Check sheet for the modelled part. Datum: model origin and axes. Units: mm. Face numbers are marked on the shaded views. A direction names the side the tool comes from. Give positions to 0.01 mm unless a question says otherwise; leave off trailing zeros. Write each loop counter-clockwise with the first axis right and the second up, starting at its lowest first coordinate (ties: lowest second). Pieces come first, ordered by that corner, then holes. Notation, with made-up numbers: M -8,11.5 L 10,11.5 A13 ccw 10,28.5 Z; hole C 33.5,-23 d2. An arc over 180 degrees is marked long. Use CSV: the item, a comma, the result in double quotes. Start each with the question number.
1. Depth check by flat-ended pin: P1, Ø2, axis at x = -4.5, z = 5, coming from the -Y side; P2, Ø4, axis at x = -3.5, z = 2.5, coming from the +Y side. Enter the tip coordinate at first touch or a pass-through.
2. Cross-section at A-A, the plane y = 0.5. Enter the section's corners in (x, z), and give its area (3 significant figures).
3. Access from +Z, -Z, +X, -X, +Y, -Y to the whole of each face (thin tool, end or side, straight path). Record for the marked faces 4 and 5.
4. Mould release check, pull along Z, two halves, no side actions. Record for the marked faces 1, 2 and 3: +Z half, -Z half, draft (parallel to the pull), parting line (faces both ways), or undercut.
5. Cross-section at D-D, the plane y = 1.25. Enter the section's corners in (x, z).
6. Cross-section at C-C, the plane z = 5.75. Enter the section's corners in (x, y), and give its area (3 significant figures).
7. Scan lines: line 1 (Z direction, x = -4.5, y = 1); line 2 (X direction, y = 2, z = 4); line 3 (Z direction, x = -6, y = 1.75). Record each from-to range of solid material in increasing order.
8. Cross-section at B-B, the plane x = -4.75. Enter the section's corners in (y, z).
from build123d import *

# Parameters (mm, degrees)
BOSS_EXTRUDE1_DEPTH = 7.8
SHELL1_T            = -1.5


with BuildPart() as part:
    # Sketch1 → Boss-Extrude1 (new body)
    with BuildSketch(Plane(origin=(0, 0, 0), x_dir=(0, 0, -1), z_dir=(1, 0, 0))):
        Polygon((0, 0), (-7.8, 0), (-7.8, 2), (0, 6.15), align=None)
    extrude(amount=-BOSS_EXTRUDE1_DEPTH)

    # Shell1
    shell1_openings = [part.faces().sort_by_distance(p)[0] for p in [
        (-3.9, 0, 3.9),
    ]]
    offset(amount=SHELL1_T, openings=shell1_openings, kind=Kind.INTERSECTION)


solid = part.part
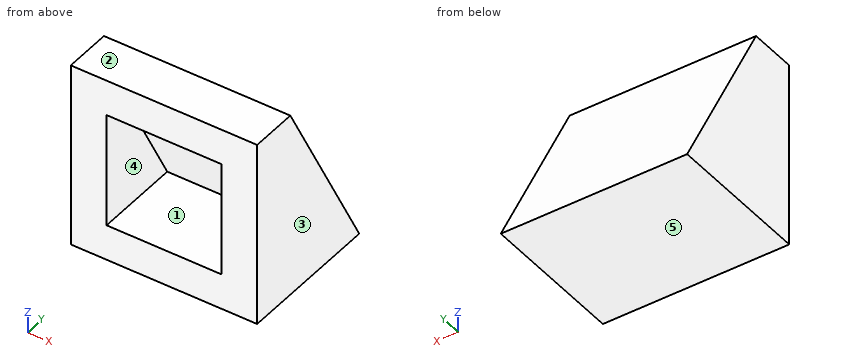
Worked answers:
1,P1,"stops at y = 1.26"
1,P2,"stops at y = 5.88"
2,outline,"M -7.8,0 L 0,0 L 0,7.8 L -7.8,7.8 Z; hole M -6.3,1.5 L -1.5,1.5 L -1.5,6.3 L -6.3,6.3 Z"
2,area,"37.8 mm^2"
3,face 4,"-Y"
3,face 5,"-Z, +X, -X, +Y, -Y"
4,face 1,"undercut"
4,face 2,"+Z half"
4,face 3,"draft"
5,outline,"M -7.8,0 L 0,0 L 0,7.8 L -7.8,7.8 Z; hole M -6.3,1.5 L -1.5,1.5 L -1.5,6.02 L -6.3,6.02 Z"
6,outline,"M -7.8,0 L -6.3,0 L -6.3,1.39 L -1.5,1.39 L -1.5,0 L 0,0 L 0,3.09 L -7.8,3.09 Z"
6,area,"17.4 mm^2"
7,line 1,"z = 0 to 1.5, 6.3 to 7.8"
7,line 2,"x = -7.8 to -6.3, -1.5 to 0"
7,line 3,"z = 0 to 1.5, 5.08 to 7.8"
8,outline,"M 0,0 L 6.15,0 L 2,7.8 L 0,7.8 L 0,6.3 L 1.1,6.3 L 3.65,1.5 L 0,1.5 Z"
